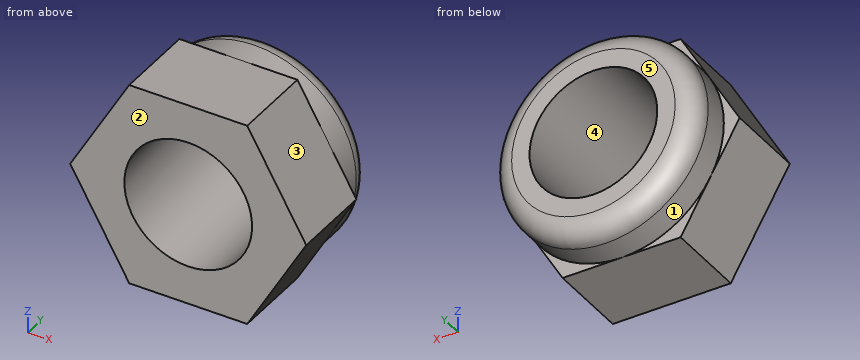
```python
from build123d import *

# Parameters (mm, degrees)
BOSS_EXTRUDE1_DEPTH = 3.2
SKETCH2_R           = 4
BOSS_EXTRUDE2_DEPTH = 1.8
SKETCH3_R           = 2.5
CUT_EXTRUDE1_DEPTH  = 8.895146188
FILLET1_R           = 0.8


with BuildPart() as part:
    # Sketch1 → Boss-Extrude1 (new body)
    with BuildSketch(Plane(origin=(0, 0, 0), x_dir=(1, 0, 0), z_dir=(0, 1, 0))):
        Polygon((4.618802154, 0), (2.309401077, 4), (-2.309401077, 4), (-4.618802154, 0), (-2.309401077, -4), (2.309401077, -4), align=None)
    extrude(amount=BOSS_EXTRUDE1_DEPTH)

    # Sketch2 → Boss-Extrude2 (add)
    with BuildSketch(Plane(origin=(0, 3.2, 0), x_dir=(1, 0, 0), z_dir=(0, 1, 0))):
        with Locations(Location((0, 0, 0), (0, 0, 270))):
            Circle(SKETCH2_R)
    extrude(amount=BOSS_EXTRUDE2_DEPTH)

    # Sketch3 → Cut-Extrude1 (cut, through all)
    with BuildSketch(Plane(origin=(0, 5, 0), x_dir=(1, 0, 0), z_dir=(0, 1, 0))):
        with Locations(Location((0, 0, 0), (0, 0, 270))):
            Circle(SKETCH3_R)
    extrude(amount=-CUT_EXTRUDE1_DEPTH, mode=Mode.SUBTRACT)

    # Fillet1
    fillet1_edges = [part.edges().sort_by_distance(p)[0] for p in [
        (0, 5, -4),
    ]]
    fillet(fillet1_edges, radius=FILLET1_R)


solid = part.part
```
Work out the finished part from the listing and answer in its coordinate system (mm). Face numbers are marked on the shaded views. A direction names the side the tool comes from. Give positions to 0.01 mm unless a question says otherwise; leave off trailing zeros. Loops run counter-clockwise (first coordinate to the right, second up) from the corner with the lowest first, then second, coordinate; pieces in that order, holes last. Notation, with made-up numbers: (-23.75, -21) -> (-14.75, -21) arc R17 ccw to (-14.75, 11) -> close; hole circle Ø8 at (40, 4.25). An arc over 180 degrees is marked (long way). Use CSV: the item, a comma, the result in double quotes.
1. Straight lines are drawn through the part: line 1 (X direction, y = 3.35, z = 0); line 2 (Z direction, x = 1.25, y = 3.3); line 3 (Z direction, x = -0.5, y = 2). For each, find the intervals that lie inside material, in ascending order.
Found:
line 1,"-4 to -2.5, 2.5 to 4"
line 2,"-3.8 to -2.17, 2.17 to 3.8"
line 3,"-4 to -2.45, 2.45 to 4"
2. Flat-ended cylindrical pins translate along their axes: pin 1 Ø0.6 at (x, z) = (-1, -3.5) entering from +Y; pin 2 Ø3 at (x, z) = (0, 0) entering from +Y; pin 3 Ø2 at (y, z) = (4, -3) entering from +X. Find the tip coordinate at first contact, or state that the pin passes through.
Found:
pin 1,"y = 4.99"
pin 2,"through"
pin 3,"x = 3.46"
3. The part is cut by section C-C (y = 4.45). Write down the section's boundary in (x, z), then the cut area to 3 significant figures.
Found:
outline,"circle Ø7.92 at (0, 0); hole circle Ø5 at (0, 0)"
area,"29.6 mm^2"
4. The part is cut by section A-A (y = 1.95). Write down the section's boundary in (x, z).
Found:
outline,"(-4.62, 0) -> (-2.31, -4) -> (2.31, -4) -> (4.62, 0) -> (2.31, 4) -> (-2.31, 4) -> close; hole circle Ø5 at (0, 0)"
5. The part is cut by section B-B (y = 3.35). Write down the section's boundary in (x, z).
Found:
outline,"circle Ø8 at (0, 0); hole circle Ø5 at (0, 0)"
6. The mould has two halves that part along X. Classify the marked faces 3, 4 and 5: +X half, -X half, draft (parallel to the pull), parting line (faces both ways), or undercut.
Found:
face 3,"+X half"
face 4,"undercut"
face 5,"draft"
7. A tool of negligible diameter and unlimited length cuts with its end or side. For the marked faces 1 and 2, from which of +Z, -Z, +X, -X, +Y, -Y can it reach the whole face along a straight path? Write none if from no direction.
Found:
face 1,"+Y"
face 2,"+Z, -Z, +X, -X, -Y"
